Geometry check sheet. Reference: the model listing, model coordinates, mm. Give positions to 0.01 mm unless a question says otherwise; leave off trailing zeros. Order: outer loops, then holes, each group sorted by start corner. A loop starts at its lowest first (then second) coordinate and runs counter-clockwise, first axis right, second up. Notation, with made-up numbers: M 36.25,-21.75 L 71.25,-21.75 A6 cw 71.25,-11.75 Z; hole C -31.75,-13.5 d1. An arc over 180 degrees is marked long. Put each result on its own line as item: value. Start each with the question number.
Q1. Material ranges on L1, parallel to Z at x = 6.25, y = -67; L2, parallel to Z at x = 4.25, y = -62.3; L3, parallel to Z at x = 0.5, y = -16, recorded low to high.
Q2. Section check D-D on z = 45.2. Record the cut outline in (x, y).
Q3. Section check B-B on z = -104.8. Record the cut outline in (x, y).
Q4. Go/stop test with flat-tipped pins: pin 1 (4 mm diameter, centred on y = 38.27, z = -77.5, fed in from -X); pin 2 (2 mm diameter, centred on x = 6, z = -71.5, fed in from -Y); pin 3 (4 mm diameter, centred on x = 5, z = 127, fed in from +Y); pin 4 (2 mm diameter, centred on x = 3.5, z = 85.5, fed in from +Y). Record where each tip stops, or that it passes through.
Q5. Section check C-C on x = 2. State how many separate pieces and enclosed holes the cut face has, then the cut area to 3 significant figures.
Q6. Section check A-A on y = 62.3. Record the cut outline in (x, z).
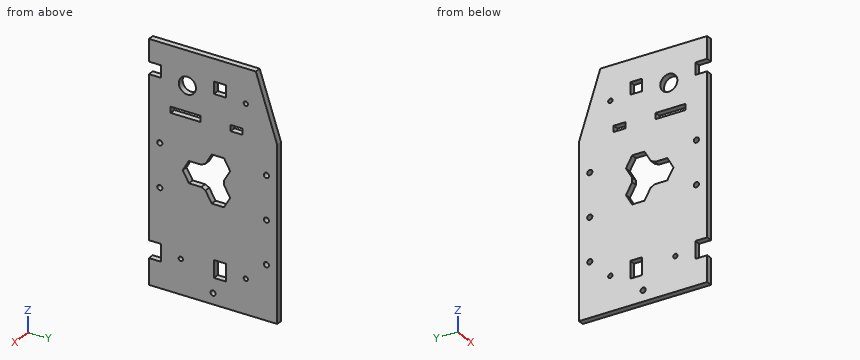
```python
from build123d import *

# Parameters (mm, degrees)
SKETCH1_R                = 10
SKETCH1_R_2              = 2.5
SKETCH1_W                = 14
SKETCH1_H                = 14
SKETCH1_W_2              = 20
SKETCH1_W_3              = 7
SKETCH1_H_2              = 35
BOSS_EXTRUDE1_DEPTH      = 7
F_6_0_6_DIAMETER_HOLE1_D = 6


with BuildPart() as part:
    # Sketch1 → Boss-Extrude1 (new body)
    with BuildSketch(Plane(origin=(0, 0, 0), x_dir=(0, 0, -1), z_dir=(1, 0, 0))):
        Polygon((-118.5, -75), (67.5, -75), (67.5, -61), (87.5, -61), (87.5, -75), (117.5, -75), (117.5, 75), (-83, 75), (-158, 50), (-158, -75), (-132.5, -75), (-132.5, -61), (-118.5, -61), align=None)
        with Locations((-118.75, -30.05)):
            Circle(SKETCH1_R, mode=Mode.SUBTRACT)
        with Locations((77.5, 38.27)):
            Circle(SKETCH1_R_2, mode=Mode.SUBTRACT)
        with Locations((-118.5, 38.27)):
            Circle(SKETCH1_R_2, mode=Mode.SUBTRACT)
        with Locations((77.5, -37.73)):
            Circle(SKETCH1_R_2, mode=Mode.SUBTRACT)
        with Locations((-125.5, 8)):
            Rectangle(SKETCH1_W, SKETCH1_H, mode=Mode.SUBTRACT)
        with Locations((77.5, 8)):
            Rectangle(SKETCH1_W_2, SKETCH1_H, mode=Mode.SUBTRACT)
        Polygon((-22.397299346, -35.516686773), (-9.948649676, -28.211588915), (-9.948649676, -13.777832185), (-7.5, -8.867513459), (5, -1.650635095), (5, 12.783121635), (-7.5, 20), (-20, 12.783121635), (-25, 12.783121635), (-37.5, 20), (-50, 12.783121635), (-50, -1.650635095), (-37.5, -8.867513459), (-34.94864967, -13.955732953), (-34.94864967, -28.389489683), align=None, mode=Mode.SUBTRACT)
        with Locations((-86, 27.4)):
            Rectangle(SKETCH1_W_3, SKETCH1_H, mode=Mode.SUBTRACT)
        with Locations((-86, -32.1)):
            Rectangle(SKETCH1_W_3, SKETCH1_H_2, mode=Mode.SUBTRACT)
    extrude(amount=BOSS_EXTRUDE1_DEPTH)

    # Ø6.0 (6) Diameter Hole1 (through all)
    with Locations(Plane(origin=(7, -62.3, -4.8), x_dir=(0, 0, 1), z_dir=(1, 0, 0))):
        with Locations((0, 0), (-100, -62.3), (-50, -124.6), (0, -124.6), (50, -124.6), (50, 0)):
            Hole(F_6_0_6_DIAMETER_HOLE1_D / 2)


solid = part.part
```
Results found:
1. L1: z = -117.5 to -87.5, -67.5 to 118.5, 132.5 to 158
1. L2: z = -117.5 to -87.5, -67.5 to -7.8, -1.8 to 42.2, 48.2 to 118.5, 132.5 to 158
1. L3: z = -117.5 to 9.95, 34.95 to 82.5, 89.5 to 158
2. outline: M 0,-75 L 7,-75 L 7,-65.3 L 0,-65.3 Z; M 0,-59.3 L 7,-59.3 L 7,-4.42 L 0,-4.42 Z; M 0,15.55 L 7,15.55 L 7,59.3 L 0,59.3 Z; M 0,65.3 L 7,65.3 L 7,75 L 0,75 Z
3. outline: M 0,-75 L 7,-75 L 7,-3 L 0,-3 Z; M 0,3 L 7,3 L 7,75 L 0,75 Z
4. pin 1: passes through
4. pin 2: stops at y = -61
4. pin 3: stops at y = 61
4. pin 4: stops at y = 74.5
5. separate pieces: 1
5. enclosed holes: 15
5. area: 36,700 mm^2
6. outline: M 0,-117.5 L 7,-117.5 L 7,-57.8 L 0,-57.8 Z; M 0,-51.8 L 7,-51.8 L 7,-7.8 L 0,-7.8 Z; M 0,-1.8 L 7,-1.8 L 7,42.2 L 0,42.2 Z; M 0,48.2 L 7,48.2 L 7,121.1 L 0,121.1 Z
